Source: CAD feature listing. Evaluate the final solid. Frame: model axes, mm. A direction names the side the tool comes from. Round coordinates to 2 decimals unless told otherwise and drop trailing zeros. Order: outer loops, then holes, each group sorted by start corner. A loop starts at its lowest first (then second) coordinate and runs counter-clockwise, first axis right, second up.
```python
from build123d import *
from OCP.BRepFilletAPI import BRepFilletAPI_MakeChamfer

# Parameters (mm, degrees)
ESBO_O1_R                  = 1
RESSALTO_EXTRUS_O1_DEPTH   = 12.5
ESBO_O2_R                  = 3.5
ESBO_O2_R_2                = 1
CORTE_EXTRUS_O1_DEPTH      = 15
CORTE_EXTRUS_O2_DEPTH      = 56.625983137
CORTE_EXTRUS_O2_DEPTH_BACK = 56.625983137
ESBO_O4_W                  = 13
ESBO_O4_H                  = 18
ESBO_O5_R                  = 1.7
RESSALTO_EXTRUS_O2_DEPTH   = 3
CHANFRO1_SIZE              = 3
CHANFRO1_SIZE2             = 4.28444402
ESBO_O7_R                  = 1.75
CORTE_EXTRUS_O3_DEPTH      = 10
CORTE_EXTRUS_O4_DEPTH      = 63.08260626
RESSALTO_EXTRUS_O3_START   = -4
RESSALTO_EXTRUS_O3_DEPTH   = 4


with BuildPart() as part:
    # Esbo_o1 → Ressalto-extrus_o1 (new, symmetric)
    with BuildSketch(Plane.XY):
        Polygon((0, -21.5), (-43, -21.5), (-43, -18.5), (-3, -18.5), (-3, 18.5), (-43, 18.5), (-43, 21.5), (0, 21.5), (13, 21.5), (13, 11.5), (0, 11.5), (0, -11.5), (13, -11.5), (13, -21.5), align=None)
        with Locations((6.5, 13.85)):
            Circle(ESBO_O1_R, mode=Mode.SUBTRACT)
        with Locations(Location((6.5, -13.85, 0), (0, 0, 180))):
            Circle(ESBO_O1_R, mode=Mode.SUBTRACT)
    extrude(amount=RESSALTO_EXTRUS_O1_DEPTH, both=True)

    # Esbo_o2 → Corte-extrus_o1 (cut)
    with BuildSketch(Plane(origin=(0, 21.5, 0), x_dir=(1, 0, 0), z_dir=(0, 1, 0))):
        with Locations(Location((-30.5, 0, 0), (0, 0, 270))):
            Circle(ESBO_O2_R)
        with Locations(Location((-14.5, 0, 0), (0, 0, 270))):
            Circle(ESBO_O2_R_2)
        with BuildLine():
            Line((-30.5, 12.5), (-64.159261009, 12.5))
            Line((-64.159261009, 12.5), (-64.159261009, -12.5))
            Line((-64.159261009, -12.5), (-30.5, -12.5))
            ThreePointArc((-30.5, -12.5), (-43, 0), (-30.5, 12.5))
        make_face()
    extrude(amount=-CORTE_EXTRUS_O1_DEPTH, mode=Mode.SUBTRACT)

    # Esbo_o4 → Corte-extrus_o2 (cut, two sides: drawn at the far end of the back side and taken through both)
    with BuildSketch(Plane(origin=(0, -11.5, 0), x_dir=(1, 0, 0), z_dir=(0, 1, 0)).offset(-CORTE_EXTRUS_O2_DEPTH_BACK)):
        with Locations((6.5, 3.5)):
            Rectangle(ESBO_O4_W, ESBO_O4_H)
    extrude(amount=CORTE_EXTRUS_O2_DEPTH + CORTE_EXTRUS_O2_DEPTH_BACK, mode=Mode.SUBTRACT)

    # Esbo_o5 → Ressalto-extrus_o2 (add)
    with BuildSketch(Plane(origin=(0, 0, -12.5), x_dir=(-1, 0, 0), z_dir=(0, 0, -1))):
        with BuildLine():
            Line((-8.182323793, 11.928517871), (0, 14.120964923))
            Line((0, 14.120964923), (0, -2.820964923))
            Line((0, -2.820964923), (-8.182323793, -0.628517871))
            ThreePointArc((-8.182323793, -0.628517871), (-13, 5.65), (-8.182323793, 11.928517871))
        make_face()
        with Locations((-6.5, 5.65)):
            Circle(ESBO_O5_R, mode=Mode.SUBTRACT)
    extrude(amount=-RESSALTO_EXTRUS_O2_DEPTH)

    # Chanfro1: one chamfer whose edges measure the first distance from different faces: ONE call of the kernel's chamfer builder (chamfer() names one face for all edges)
    chanfro1_edges_1 = [part.edges().sort_by_distance(p)[0] for p in [
        (-3, 18.5, 0),
    ]]
    chanfro1_side_1 = [part.faces().sort_by_distance(p)[0] for p in [
        (-21.411390312, 18.5, 0),
    ]]
    chanfro1_edges_2 = [part.edges().sort_by_distance(p)[0] for p in [
        (-3, -18.5, 0),
    ]]
    chanfro1_side_2 = [part.faces().sort_by_distance(p)[0] for p in [
        (-23, -18.5, 0),
    ]]
    chanfro1 = BRepFilletAPI_MakeChamfer(part.part.solid().wrapped)
    for e in chanfro1_edges_1:
        chanfro1.Add(CHANFRO1_SIZE, CHANFRO1_SIZE2, e.wrapped, chanfro1_side_1[0].wrapped)  # the first distance lies on this face
    for e in chanfro1_edges_2:
        chanfro1.Add(CHANFRO1_SIZE, CHANFRO1_SIZE2, e.wrapped, chanfro1_side_2[0].wrapped)  # the first distance lies on this face
    add(Compound.cast(chanfro1.Shape()), mode=Mode.REPLACE)

    # Esbo_o7 → Corte-extrus_o3 (cut)
    with BuildSketch(Plane(origin=(0, -18.5, 0), x_dir=(1, 0, 0), z_dir=(0, 1, 0))):
        with Locations(Location((-30.5, 0, 0), (0, 0, 270))):
            Circle(ESBO_O7_R)
    extrude(amount=-CORTE_EXTRUS_O3_DEPTH, mode=Mode.SUBTRACT)

    # Esbo_o2_2 → Corte-extrus_o4 (cut, through all)
    with BuildSketch(Plane(origin=(0, 21.5, 0), x_dir=(1, 0, 0), z_dir=(0, 1, 0))):
        Polygon((-43, -3e-08), (-43, 12.5), (-64.159261009, 12.5), (-64.159261009, -12.5), (-43, -12.5), align=None)
        with BuildLine():
            ThreePointArc((-30.5, -12.5), (-39.338834754, -8.838834775), (-43, -3e-08))
            Line((-43, -3e-08), (-43, -12.5))
            Line((-43, -12.5), (-30.5, -12.5))
        make_face()
        with BuildLine():
            ThreePointArc((-43, -3e-08), (-39.338834775, 8.838834754), (-30.5, 12.5))
            Line((-30.5, 12.5), (-43, 12.5))
            Line((-43, 12.5), (-43, -3e-08))
        make_face()
    extrude(amount=-CORTE_EXTRUS_O4_DEPTH, mode=Mode.SUBTRACT)

    # Esbo_o8 → Ressalto-extrus_o3 (add)
    with BuildSketch(Plane(origin=(0, 0, 0), x_dir=(0, 0, -1), z_dir=(1, 0, 0)).offset(RESSALTO_EXTRUS_O3_START)):
        Polygon((-10, 21.5), (-3, 28.5), (7, 28.5), (7, 25.5), (5, 24), (5, 25.5), (-1.757359313, 25.5), (-5.757359313, 21.5), align=None)
    extrude(amount=-RESSALTO_EXTRUS_O3_DEPTH)


solid = part.part
```
1. Pull-direction query (X, two-part tool) for faces 1 (the face through (-4, 26, 1)), 2 (the face through (-28.765, -19.979, -0.228)), 3 (the face through (-5.972, 24.76, -6.014)); classes: released by +X, released by -X, zero draft, split by the parting line, or undercut.
2. First-contact query: pin 1 (3 mm diameter, centred on x = -14.5, z = 0, fed in from +Y); pin 2 (4 mm diameter, centred on x = 5, y = 4.5, fed in from +Z); pin 3 (8 mm diameter, centred on x = 6, y = -16, fed in from -Z). Flat tips, straight axial feed; report the tip coordinate or a pass-through.
3. Section A-A on x = -14.5. Return loops of the section in (y, z).
4. Section C-C on x = 6.5. Return loops of the section in (y, z), plus the area to 3 significant figures.
5. Line query: line 1 along X through (y, z) = (20.85, 0); line 2 along Y through (x, z) = (6.5, 9); line 3 along Y through (x, z) = (-9.5, 3.5). Output: solid intervals per line, ascending.
6. Access query for faces 4 (the face through (-27, 20, 0)), 5 (the face through (-4.48, 16.33, 0.17)), 6 (the face through (-6, 25, -5)). Directions: +Z, -Z, +X, -X, +Y, -Y. A direction counts if a zero-diameter tool reaches every point of the face in a straight line with its end or side. Return the directions, or none.
7. Section B-B on y = 5.65. Return loops of the section in (x, z), plus the area to 3 significant figures.
8. Section D-D on z = 8. Return loops of the section in (x, y), plus the area to 3 significant figures.
Result:
1. face 1: released by +X
1. face 2: undercut
1. face 3: zero draft
2. pin 1: stops at y = 21.5
2. pin 2: stops at z = -9.5
2. pin 3: stops at z = 5.5
3. outline: (-21.5, -12.5) - (-18.5, -12.5) - (-18.5, 12.5) - (-21.5, 12.5) - close; (18.5, -12.5) - (21.5, -12.5) - (21.5, -1) - (18.5, -1) - close; (18.5, 1) - (21.5, 1) - (21.5, 12.5) - (18.5, 12.5) - close
4. outline: (-21.5, 5.5) - (-14.85, 5.5) - (-14.85, 12.5) - (-21.5, 12.5) - close; (-12.85, 5.5) - (-11.5, 5.5) - (-11.5, 12.5) - (-12.85, 12.5) - close; (-1.08, -12.5) - (3.95, -12.5) - (3.95, -9.5) - (-1.08, -9.5) - close; (7.35, -12.5) - (12.38, -12.5) - (12.38, -9.5) - (7.35, -9.5) - close; (11.5, 5.5) - (12.85, 5.5) - (12.85, 12.5) - (11.5, 12.5) - close; (14.85, 5.5) - (21.5, 5.5) - (21.5, 12.5) - (14.85, 12.5) - close
4. area: 142 mm2
5. line 1: x = -43 to -34, -27 to -15.5, -13.5 to 0
5. line 2: y = -21.5 to -14.85, -12.85 to -11.5, 11.5 to 12.85, 14.85 to 21.5
5. line 3: y = -21.5 to -18.5, 18.5 to 21.5
6. face 4: +Y
6. face 5: +Z, -Z, -X
6. face 6: +X, -X
7. outline: (-3, -12.5) - (4.8, -12.5) - (4.8, -9.5) - (0, -9.5) - (0, 12.5) - (-3, 12.5) - close; (8.2, -12.5) - (13, -12.5) - (13, -9.5) - (8.2, -9.5) - close
7. area: 104 mm2
8. outline: (-40.1, -21.5) - (13, -21.5) - (13, -11.5) - (0, -11.5) - (0, 11.5) - (13, 11.5) - (13, 21.5) - (-4, 21.5) - (-4, 23.5) - (-8, 23.5) - (-8, 21.5) - (-40.1, 21.5) - (-40.1, 18.5) - (-6, 18.5) - (-3, 14.22) - (-3, -14.22) - (-6, -18.5) - (-40.1, -18.5) - close; hole circle Ø2 at (6.5, -13.85); hole circle Ø2 at (6.5, 13.85)
8. area: 626 mm2
